from build123d import *

# Parameters (mm, degrees)
F1_DEPTH  = 152.4
F3_DEPTH  = 154.432
F4_W      = 32.220531255
F4_H      = 154.432
F5_DEPTH  = 3
F6_R      = 7.5954813499
F6_R_2    = 5.3319461193
F7_DEPTH  = 2
F9_DEPTH  = 12
F10_W     = 112.0086535811
F10_H     = 112.0086535811
F11_DEPTH = 25.4


with BuildPart() as f1:
    # F0 (on Top) → F1 (new body)
    with BuildSketch(Plane.XY):
        with BuildLine():
            Line((-134.2638241291, 0), (0, 0))
            Line((0, 0), (22.4686227739, 0))
            Line((22.4686227739, 0), (22.4686227739, 6.3499999233))
            Line((22.4686227739, 6.3499999233), (0, 6.3499999233))
            Line((0, 6.35), (-128.7519809926, 6.35))
            ThreePointArc((-128.7519809926, 6.35), (-131.8256525814, 7.9086353107), (-132.3845036601, 11.3092950319))
            Line((-132.3845036601, 11.3092950319), (-94.8052258673, 130.0843481086))
            ThreePointArc((-94.8052258673, 130.0843481086), (-93.4240678892, 132.0087246655), (-91.1727031999, 132.7450530767))
            Line((-91.1727031999, 132.7450530767), (-24.7038652326, 132.7450530767))
            ThreePointArc((-24.7038652326, 132.7450530767), (-22.2165192123, 131.8210901131), (-20.9355855807, 129.4973416727))
            Line((-20.9355855807, 129.4973416727), (-7.0881516681, 36.6962359353))
            ThreePointArc((-7.0881516681, 36.6962359353), (-2.8183728961, 28.9504078005), (5.4727805049, 25.870531255))
            Line((5.4727805049, 25.870531255), (22.4686227739, 25.870531255))
            Line((22.4686227739, 25.870531255), (22.4686227739, 32.220531255))
            Line((22.4686227739, 32.220531255), (5.4727805049, 32.220531255))
            ThreePointArc((5.4727805049, 32.220531255), (1.3272038044, 33.7604695277), (-0.8076855816, 37.6333835952))
            Line((-0.8076855816, 37.6333835952), (-15.1397308432, 133.6822007366))
            ThreePointArc((-15.1397308432, 133.6822007366), (-17.2746202291, 137.555114804), (-21.4201969297, 139.0950530767))
            Line((-21.4201969297, 139.0950530767), (-93.9634045544, 139.0950530767))
            ThreePointArc((-93.9634045544, 139.0950530767), (-97.7156790366, 137.867839058), (-100.0176090002, 134.6605447965))
            Line((-100.0176090002, 134.6605447965), (-140.6138241291, 6.35))
            ThreePointArc((-140.6138241291, 6.35), (-138.7539521896, 1.8598719395), (-134.2638241291, 0))
        make_face()
    extrude(amount=F1_DEPTH)

    # F2 (on face) → F3 (join)
    with BuildSketch(Plane.XY.offset(152.4)):
        with BuildLine():
            Line((-134.2638241291, 0), (0, 0))
            Line((0, 0), (22.4686227739, 0))
            Line((22.4686227739, 0), (22.4686227739, 13.6102656275))
            Line((22.4686227739, 13.6102656275), (17.4686227739, 13.6102656275))
            Line((17.4686227739, 13.6102656275), (17.4686227739, 18.6102656275))
            Line((17.4686227739, 18.6102656275), (22.4686227739, 18.6102656275))
            Line((22.4686227739, 18.6102656275), (22.4686227739, 32.220531255))
            Line((22.4686227739, 32.220531255), (5.4727805049, 32.220531255))
            ThreePointArc((5.4727805049, 32.220531255), (1.3272038044, 33.7604695277), (-0.8076855816, 37.6333835952))
            Line((-0.8076855816, 37.6333835952), (-15.1397308432, 133.6822007366))
            ThreePointArc((-15.1397308432, 133.6822007366), (-17.2746202291, 137.555114804), (-21.4201969297, 139.0950530767))
            Line((-21.4201969297, 139.0950530767), (-93.9634045544, 139.0950530767))
            ThreePointArc((-93.9634045544, 139.0950530767), (-97.7156790366, 137.867839058), (-100.0176090002, 134.6605447965))
            Line((-100.0176090002, 134.6605447965), (-140.6138241291, 6.35))
            ThreePointArc((-140.6138241291, 6.35), (-138.7539521896, 1.8598719395), (-134.2638241291, 0))
        make_face()
    extrude(amount=-F3_DEPTH)

    # F4 (on face) → F5 (join)
    with BuildSketch(Plane.YZ.offset(22.4686227739)):
        with Locations((16.1102656275, 75.184)):
            Rectangle(F4_W, F4_H)
    extrude(amount=F5_DEPTH)

    # F6 (on face) → F7 (join)
    with BuildSketch(Plane.YZ.offset(25.4686227739)):
        with Locations((16.0748194903, 13.0553431809)):
            Circle(F6_R)
        with Locations((15.8114936203, 52.0275905728)):
            Circle(F6_R_2)
        with Locations((15.8114936203, 70.9870681167)):
            Circle(F6_R_2)
    extrude(amount=F7_DEPTH)

    # F8 (on face) → F9 (cut)
    with BuildSketch(Plane.YZ.offset(25.4686227739)):
        with BuildLine():
            Line((17.7747905254, 142.1712523777), (15.1247905254, 142.1712523777))
            Line((15.1247905254, 142.1712523777), (15.1247905254, 116.7472228408))
            Line((15.1247905254, 116.7472228408), (17.7747905254, 116.7472228408))
            ThreePointArc((17.7747905254, 116.7472228408), (22.264918586, 118.6070947803), (24.1247905254, 123.0972228408))
            Line((24.1247905254, 123.0972228408), (24.1247905254, 135.8212523777))
            ThreePointArc((24.1247905254, 135.8212523777), (22.264918586, 140.3113804383), (17.7747905254, 142.1712523777))
        make_face()
    extrude(amount=-F9_DEPTH, mode=Mode.SUBTRACT)

    # F10 (on face) → F11 (cut)
    with BuildSketch(Plane(origin=(-129.6450638104, 41.0184440351, 0), x_dir=(-0.3016522393, -0.953418023, 0), z_dir=(-0.953418023, 0.3016522393, 0))):
        with Locations((-29.8443771899, 75.3790028393)):
            Rectangle(F10_W, F10_H)
    extrude(amount=-F11_DEPTH, mode=Mode.SUBTRACT)


solid = f1.part
Work out the finished part from the listing and answer in its coordinate system (mm). A direction names the side the tool comes from. Give positions to 0.01 mm unless a question says otherwise; leave off trailing zeros. Write each loop counter-clockwise with the first axis right and the second up, starting at its lowest first coordinate (ties: lowest second). Pieces come first, ordered by that corner, then holes. Notation, with made-up numbers: M -5,69 L -1,69 A15 cw -1,79 Z; hole C 77,-4.5 d10. An arc over 180 degrees is marked long. Answer as CSV lines item,"result".
Q1. Given P1, Ø5, axis at y = 27, z = 95.5, coming from the -X side; P2, Ø10, axis at x = 14, z = 43.5, coming from the +Y side; P3, Ø6, axis at y = 57, z = 133, coming from the +X side, each flat-ended and moving along its own axis, determine where each tip first touches the part or whether it passes through.
A:
P1,"stops at x = -108.23"
P2,"stops at y = 32.22"
P3,"stops at x = -3.25"
Q2. A cutting plane is placed at C-C on x = -107. Write down the section's boundary in (y, z).
A:
outline,"M 0,-2.03 L 112.59,-2.03 L 112.59,19.37 L 28.39,19.37 L 28.39,131.38 L 112.59,131.38 L 112.59,152.4 L 0,152.4 Z"
Q3. Find the intervals of material crossed by probe 1 along Z at (x, y) = (-111, 98.5); probe 2 along X at (y, z) = (41, 143.5); probe 3 along X at (y, z) = (75, 138.5), in increasing order. Write a range as [from, to].
A:
probe 1,"z = [-2.03, 19.37], [131.38, 152.4]"
probe 2,"x = [-129.65, -1.31]"
probe 3,"x = [-118.89, -6.38]"
Q4. A cutting plane is placed at A-A on z = 38. Write down the section's boundary in (x, y), plus the area to 3 significant figures.
A:
outline,"M -140.61,6.35 A6.35 ccw -134.26,0 L 25.47,0 L 25.47,32.22 L 5.47,32.22 A6.35 cw -0.81,37.63 L -15.14,133.68 A6.35 ccw -21.42,139.1 L -93.96,139.1 A6.35 ccw -100.02,134.66 L -103.75,122.87 L -79.53,115.21 L -113.32,8.42 L -137.54,16.08 Z; hole M 17.47,13.61 L 22.47,13.61 L 22.47,18.61 L 17.47,18.61 Z"
area,"13,900 mm²"
Q5. A tool of negligible diameter and unlimited length cuts with its end or side. For faces 1 (the flat face through (-91.81, 119.09, 74.59)), 2 (the flat face through (20, 18.61, 58)), 3 (the flat face through (-125.6, 12.3, 74.6)), from which of +Z, -Z, +X, -X, +Y, -Y can it reach the whole face along a straight path? Write none if from no direction.
A:
face 1,"-X"
face 2,"+Z, -Z"
face 3,"+Y"
Q6. A cutting plane is placed at B-B on y = 77. Write down the section's boundary in (x, z), plus the area to 3 significant figures.
A:
outline,"M -118.26,-2.03 L -6.68,-2.03 L -6.68,152.4 L -118.26,152.4 L -118.26,131.38 L -91.62,131.38 L -91.62,19.37 L -118.26,19.37 Z"
area,"14,200 mm²"
Q7. The mould has two halves that part along X. Classify faces 4 (the flat face through (-56, 0, 74)), 5 (the flat face through (17.469, 16, 76)), 6 (the flat face through (27.469, 16, 13)): +X half, -X half, draft (parallel to the pull), parting line (faces both ways), or undercut.
A:
face 4,"draft"
face 5,"undercut"
face 6,"+X half"
Q8. A cutting plane is placed at D-D on z = 138. Write down the section's boundary in (x, y), plus the area to 3 significant figures.
A:
outline,"M -140.61,6.35 A6.35 ccw -134.26,0 L 25.47,0 L 25.47,15.12 L 22.47,15.12 L 22.47,13.61 L 17.47,13.61 L 17.47,15.12 L 13.47,15.12 L 13.47,23.74 L 25.47,23.74 L 25.47,32.22 L 5.47,32.22 A6.35 cw -0.81,37.63 L -15.14,133.68 A6.35 ccw -21.42,139.1 L -93.96,139.1 A6.35 ccw -100.02,134.66 Z"
area,"16,600 mm²"
